from build123d import *

# Parameters (mm, degrees)
F0_W     = 288.925
F0_H     = 1008.0625
F1_DEPTH = 19.05
F2_W     = 19.05
F2_H     = 1008.0625
F3_DEPTH = 6.35
F5_DEPTH = 6.35
F6_W     = 3.175
F6_H     = 19.05
F7_DEPTH = 288.926


with BuildPart() as f1:
    # F0 (on Right) → F1 (new body)
    with BuildSketch(Plane.YZ):
        Rectangle(F0_W, F0_H)
    extrude(amount=F1_DEPTH)

    # F2 (on face) → F3 (cut)
    with BuildSketch(Plane.YZ.offset(19.05)):
        with Locations((-84.1375, 0)):
            Rectangle(F2_W, F2_H)
        with Locations((84.1375, 0)):
            Rectangle(F2_W, F2_H)
    extrude(amount=-F3_DEPTH, mode=Mode.SUBTRACT)

    # F4 (on face) → F5 (cut)
    with BuildSketch(Plane(origin=(0, 0, 0), x_dir=(0, -1, 0), z_dir=(-1, 0, 0))):
        Polygon((93.6625, -377.03125), (93.6625, 504.03125), (74.6125, 504.03125), (74.6125, -377.03125), (74.6125, -504.03125), (93.6625, -504.03125), align=None)
        Polygon((-74.6125, 504.03125), (-93.6625, 504.03125), (-93.6625, -377.03125), (-93.6625, -504.03125), (-74.6125, -504.03125), (-74.6125, -377.03125), align=None)
    extrude(amount=-F5_DEPTH, mode=Mode.SUBTRACT)

    # F6 (on face) → F7 (cut, through all)
    with BuildSketch(Plane.XZ.offset(144.4625)):
        with Locations((1.5875, -386.55625)):
            Rectangle(F6_W, F6_H)
        with Locations((17.4625, -386.55625)):
            Rectangle(F6_W, F6_H)
    extrude(amount=-F7_DEPTH, mode=Mode.SUBTRACT)


solid = f1.part
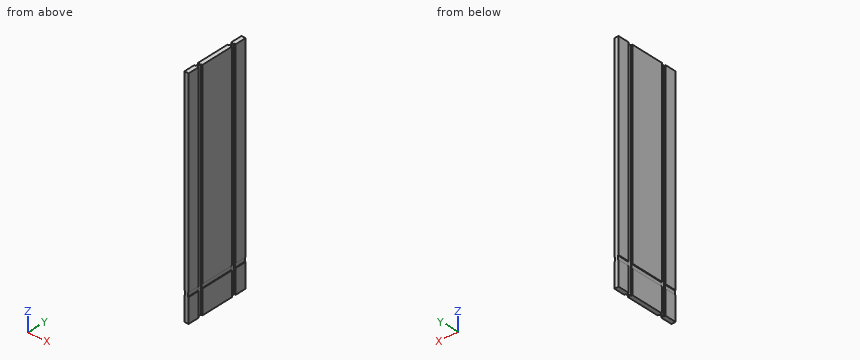
Design review of the part built by this model. Coordinates are the model's own, in mm. Coordinates: 2 decimals unless noted, no trailing zeros. Order: outer loops, then holes, each group sorted by start corner. A loop starts at its lowest first (then second) coordinate and runs counter-clockwise, first axis right, second up. Notation, with made-up numbers: (11, 69.5) - (67, 69.5) arc R34 ccw to (67, 103.5) - close; hole circle Ø4 at (-37.75, 17). An arc over 180 degrees is marked (long way). Put each result on its own line as item: value.
1) Wall thickness on L1, parallel to Y at x = 5.25, z = 151.5; L2, parallel to Z at x = 18.5, y = 12.5; L3, parallel to X at y = 80, z = -81.5: over which ranges is each line inside the solid? List them lowest first. Write a range as from..to.
Response values:
L1: y = -144.46..-93.66, -74.61..74.61, 93.66..144.46
L2: z = -504.03..-396.08, -377.03..504.03
L3: x = 6.35..12.7
2) Insertion check: P1, Ø21, axis at y = -106.5, z = -391, coming from the -X side; P2, Ø5.5, axis at y = 4, z = -385.5, coming from the +X side (3 decimals); P3, Ø9.5, axis at y = -8.5, z = -383.5, coming from the -X side (3 decimals). Each pin has a flat end and moves straight along its axis. Give the tip position at first contact, or say it passes through.
Response values:
P1: stops at x = 0
P2: stops at x = 15.875
P3: stops at x = 3.175
3) Take a section at A-A, the plane z = 330.5. Give the boundary of the cut face in (x, y), and give its area (3 significant figures).
Response values:
outline: (0, -144.46) - (19.05, -144.46) - (19.05, -93.66) - (12.7, -93.66) - (12.7, -74.61) - (19.05, -74.61) - (19.05, 74.61) - (12.7, 74.61) - (12.7, 93.66) - (19.05, 93.66) - (19.05, 144.46) - (0, 144.46) - (0, 93.66) - (6.35, 93.66) - (6.35, 74.61) - (0, 74.61) - (0, -74.61) - (6.35, -74.61) - (6.35, -93.66) - (0, -93.66) - close
area: 5,020 mm²
